Source: CAD feature listing. Evaluate the final solid. Frame: model axes, mm. Face numbers are marked on the shaded views. A direction names the side the tool comes from. Coordinates: 2 decimals unless noted, no trailing zeros. Loops run counter-clockwise (first coordinate to the right, second up) from the corner with the lowest first, then second, coordinate; pieces in that order, holes last.
Item 1: Reachability of the marked faces 1, 2 and 3 from +Z, -Z, +X, -X, +Y, -Y: full face, straight path, thin tool, end or side. Return the list, or none.
Item 2: Pin query (flat end, axial travel): pin 1 Ø10 at (x, z) = (-32.5, 28) entering from +Y; pin 2 Ø10 at (x, y) = (-15, -41) entering from +Z; pin 3 Ø20 at (x, y) = (-11, -111.5) entering from +Z; pin 4 Ø1 at (y, z) = (-93, 37.5) entering from +X. Return the tip coordinate at first contact, or that it passes through.
Item 3: Line query: probe 1 along X at (y, z) = (-40.5, 14); probe 2 along Y at (x, z) = (-8, 29.5); probe 3 along X at (y, z) = (-13, 7.5). Output: solid intervals per line, ascending.
Item 4: Section query A-A, the plane z = 21. Return the cut outline in (x, y).
Item 5: Pull-direction query (Y, two-part tool) for the marked faces 4, 5 and 6; classes: +Y half, -Y half, draft (parallel to the pull), parting line (faces both ways), or undercut.
Item 6: Section query C-C, the plane y = -52.5. Return the cut outline in (x, z), then the cut area to 3 significant figures.
Item 7: Section query D-D, the plane z = 58.5. Return the cut outline in (x, y), then the cut area to 3 significant figures.
Item 8: Section query B-B, the plane x = -6.5. Return the cut outline in (y, z).
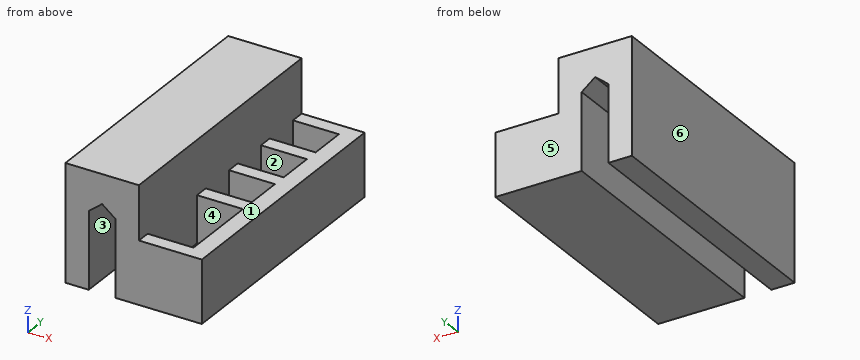
```python
from build123d import *

# Parameters (mm, degrees)
F0_W     = 0.026536879
F0_H     = 8.3333357554
F0_W_2   = 14.573463121
F1_DEPTH = 142.24
F2_W     = 27.8897660319
F2_H     = 8.4373559803
F3_DEPTH = 2.54
F4_W     = 25
F4_H     = 7.62
F5_DEPTH = 25.4


with BuildPart() as f1:
    # F0 (on Front) → F1 (new body)
    with BuildSketch(Plane.XZ):
        Polygon((-54.4296333165, 41.6801715141), (-54.4296333165, 16.0493828058), (-67.1296333165, 16.0493828058), (-67.1296333165, 0), (-54.4030964375, 0), (-54.4030964375, 41.7011594015), align=None)
        Polygon((-67.1296333165, 16.0493828058), (-54.4296333165, 16.0493828058), (-54.4296333165, 41.6801715141), (-67.1296333165, 31.6358038057), align=None)
        Polygon((-67.1296333165, 31.6358038057), (-54.4296333165, 41.6801715141), (-54.4296333165, 53.2272399031), (-56.5930453334, 54.9382718561), (-67.1296333165, 54.9382718561), align=None)
        Polygon((-54.4296333165, 53.2272399031), (-54.4296333165, 41.6801715141), (-54.4030964375, 41.7011594015), (-54.4030964375, 53.2062520157), align=None)
        Polygon((-56.5930453334, 54.9382718561), (-54.4296333165, 53.2272399031), (-54.4296333165, 54.9382718561), align=None)
        Polygon((-54.4296333165, 54.9382718561), (-54.4296333165, 53.2272399031), (-54.4030964375, 53.2062520157), (-54.4030964375, 54.9382718561), align=None)
        Polygon((-54.4030964375, 53.2062520157), (-54.4030964375, 41.7011594015), (-47.1296333165, 47.4537057086), align=None)
        Polygon((-67.1296333165, 63.2716076115), (-67.1296333165, 54.9382718561), (-56.5930453334, 54.9382718561), align=None)
        Polygon((-56.5930453334, 54.9382718561), (-54.4296333165, 54.9382718561), (-54.4296333165, 63.2716076115), (-67.1296333165, 63.2716076115), align=None)
        with Locations((-54.416364877, 59.1049397338)):
            Rectangle(F0_W, F0_H)
        Polygon((-54.4030964375, 54.9382718561), (-54.4030964375, 53.2062520157), (-47.1296333165, 47.4537057086), (-39.8296333165, 53.2272399031), (-39.8296333165, 54.9382718561), align=None)
        Polygon((-39.8296333165, 53.2272399031), (-47.1296333165, 47.4537057086), (-39.8296333165, 41.6801715141), align=None)
        with Locations((-47.116364877, 59.1049397338)):
            Rectangle(F0_W_2, F0_H)
        Polygon((-37.6662212996, 54.9382718561), (-39.8296333165, 53.2272399031), (-39.8296333165, 41.6801715141), (-27.1296333165, 31.6358038057), (-27.1296333165, 54.9382718561), align=None)
        Polygon((-39.8296333165, 54.9382718561), (-39.8296333165, 53.2272399031), (-37.6662212996, 54.9382718561), align=None)
        Polygon((-27.1296333165, 31.6358038057), (-39.8296333165, 41.6801715141), (-39.8296333165, 8.6419750216), (-39.8296333165, 0), (-27.1296333165, 0), (-27.1296333165, 8.6419750216), align=None)
        Polygon((-39.8296333165, 63.2716076115), (-39.8296333165, 54.9382718561), (-37.6662212996, 54.9382718561), (-27.1296333165, 63.2716076115), align=None)
        Polygon((-27.1296333165, 63.2716076115), (-37.6662212996, 54.9382718561), (-27.1296333165, 54.9382718561), align=None)
        Polygon((-2.1296333165, 8.6419750216), (-27.1296333165, 8.6419750216), (-27.1296333165, 0), (-2.1296333165, 0), (-2.1296333165, 1.0219750216), align=None)
        Polygon((-2.1296333165, 34.0419750216), (-2.1296333165, 8.6419750216), (-2.1296333165, 1.0219750216), (-2.1296333165, 0), (7.1296278669, 0), (7.1296278669, 1.0219750216), (7.1296278669, 34.0419750216), align=None)
    extrude(amount=F1_DEPTH)

    # F2 (on face) → F3 (join)
    with BuildSketch(Plane.XZ.offset(142.24)):
        with Locations((-25.8847503005, 4.2186779901)):
            Rectangle(F2_W, F2_H)
    extrude(amount=-F3_DEPTH)

    # F4 (on face) → F5 (join)
    with BuildSketch(Plane.XY.offset(8.6419750216)):
        with Locations((-14.6296333165, -87.63)):
            Rectangle(F4_W, F4_H)
        with Locations((-14.6296333165, -59.69)):
            Rectangle(F4_W, F4_H)
        with Locations((-14.6296333165, -31.75)):
            Rectangle(F4_W, F4_H)
        with Locations((-14.6296333165, -3.81)):
            Rectangle(F4_W, F4_H)
        Polygon((-2.1296333165, -139.7), (-2.1296333165, -134.62), (-27.1296333165, -134.62), (-27.1296333165, -142.24), (-2.1296333165, -142.24), align=None)
    extrude(amount=F5_DEPTH)


solid = f1.part
```
Verdict:
1. face 1: +Z, +X, +Y, -Y
1. face 2: +Z
1. face 3: -Z, +Y, -Y
2. pin 1: stops at y = 0
2. pin 2: stops at z = 8.64
2. pin 3: stops at z = 34.04
2. pin 4: stops at x = -27.13
3. probe 1: x = -67.13 to -54.4, -39.83 to -27.13, -2.13 to 7.13
3. probe 2: y = -142.24 to -134.62, -91.44 to -83.82, -63.5 to -55.88, -35.56 to -27.94, -7.62 to 0
3. probe 3: x = -67.13 to -54.4, -39.83 to 7.13
4. outline: (-67.13, -142.24) - (-54.4, -142.24) - (-54.4, 0) - (-67.13, 0) - close; (-39.83, -142.24) - (7.13, -142.24) - (7.13, 0) - (-39.83, 0) - close; hole (-27.13, -134.62) - (-2.13, -134.62) - (-2.13, -91.44) - (-27.13, -91.44) - close; hole (-27.13, -83.82) - (-2.13, -83.82) - (-2.13, -63.5) - (-27.13, -63.5) - close; hole (-27.13, -55.88) - (-2.13, -55.88) - (-2.13, -35.56) - (-27.13, -35.56) - close; hole (-27.13, -27.94) - (-2.13, -27.94) - (-2.13, -7.62) - (-27.13, -7.62) - close
5. face 4: undercut
5. face 5: +Y half
5. face 6: draft
6. outline: (-67.13, 0) - (-54.4, 0) - (-54.4, 41.7) - (-47.13, 47.45) - (-39.83, 41.68) - (-39.83, 0) - (7.13, 0) - (7.13, 34.04) - (-2.13, 34.04) - (-2.13, 8.64) - (-27.13, 8.64) - (-27.13, 63.27) - (-67.13, 63.27) - close
6. area: 2,410 mm2
7. outline: (-67.13, -142.24) - (-27.13, -142.24) - (-27.13, 0) - (-67.13, 0) - close
7. area: 5,690 mm2
8. outline: (-142.24, 0) - (0, 0) - (0, 34.04) - (-7.62, 34.04) - (-7.62, 8.64) - (-27.94, 8.64) - (-27.94, 34.04) - (-35.56, 34.04) - (-35.56, 8.64) - (-55.88, 8.64) - (-55.88, 34.04) - (-63.5, 34.04) - (-63.5, 8.64) - (-83.82, 8.64) - (-83.82, 34.04) - (-91.44, 34.04) - (-91.44, 8.64) - (-134.62, 8.64) - (-134.62, 34.04) - (-142.24, 34.04) - close
